Here's the drawing with two shaded views (mm, measured from the low corner). I have some questions. A direction names the side the tool comes from. Give positions to 0.01 mm unless a question says otherwise; leave off trailing zeros. Write each loop counter-clockwise with the first axis right and the second up, starting at its lowest first coordinate (ties: lowest second). Pieces come first, ordered by that corner, then holes.
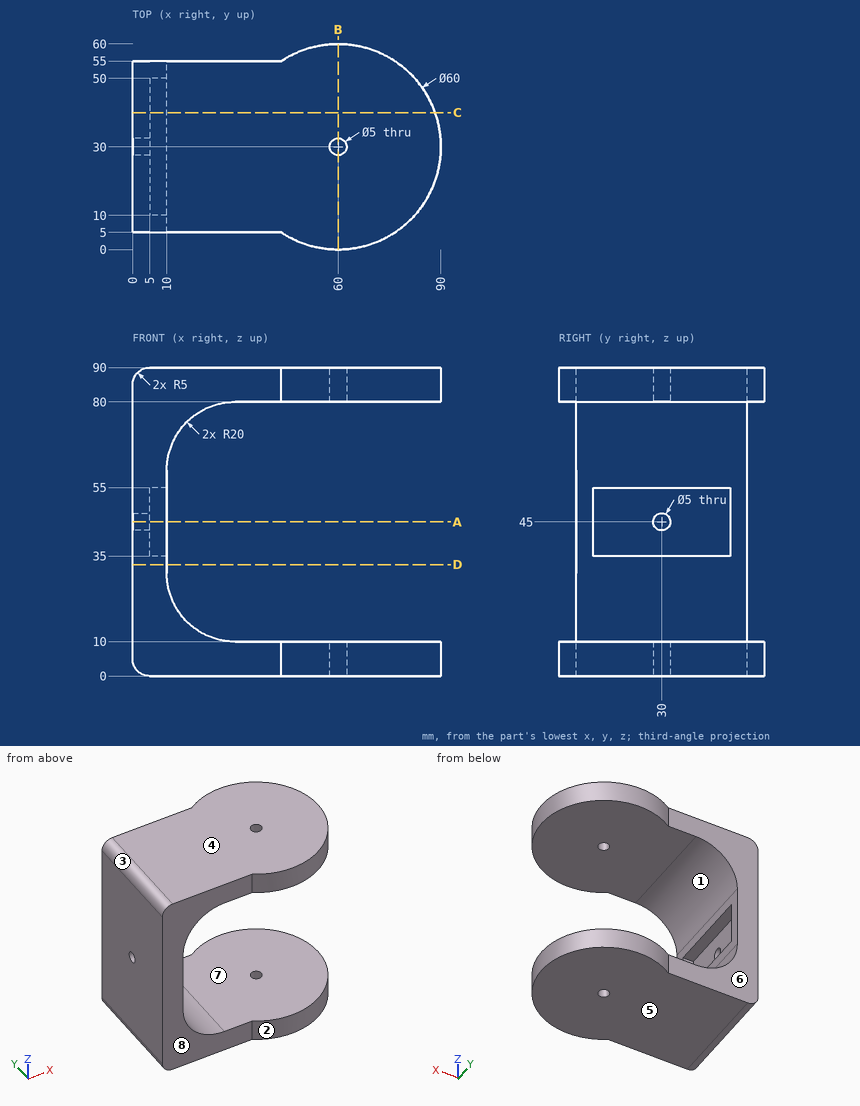
(1) Will these pins go through, and if not, where does the flat tip stop? P1, Ø22, axis at y = 34, z = 46, coming from the +X side; P2, Ø5.5, axis at x = 8, z = 42.5, coming from the -Y side; P3, Ø12, axis at x = 42, z = 11, coming from the -Y side.
Returned:
P1: stops at x = 10
P2: stops at y = 5
P3: stops at y = 2.54
(2) Imagine slicing it at B-B, the plane x = 60. Write out the boundary of the cut face in (y, z).
Returned:
outline: (0, 0) - (27.5, 0) - (27.5, 10) - (0, 10) - close; (0, 80) - (27.5, 80) - (27.5, 90) - (0, 90) - close; (32.5, 0) - (60, 0) - (60, 10) - (32.5, 10) - close; (32.5, 80) - (60, 80) - (60, 90) - (32.5, 90) - close
(3) Imagine slicing it at D-D, the plane z = 32.5. Write out the boundary of the cut face in (x, y).
Returned:
outline: (0, 5) - (10, 5) - (10, 55) - (0, 55) - close
(4) For the marked faces 4, 5, 6, 7 and 8, which set-ups out of +Z, -Z, +X, -X, +Y, -Y let a thin tool reach every point of the face, with its end or its side?
Returned:
face 4: +Z, +X, -X, +Y, -Y
face 5: -Z, +X, -X, +Y, -Y
face 6: +Z, -Z, -X, +Y
face 7: +X, +Y, -Y
face 8: +Z, -Z, -X, -Y
(5) If we mould it in two halves opening along Z, with no side actions, what happens to the marked faces 1, 2 and 3? For each: +Z half, -Z half, draft (parallel to the pull), parting line (faces both ways), or undercut.
Returned:
face 1: undercut
face 2: draft
face 3: +Z half
(6) If I drill on L1, parallel to Z at x = 67, y = 32; L2, parallel to Y at x = 2, z = 45; L3, parallel to Y at x = 60, z = 83, over which ranges is the centre line in solid material (lowest first)?
Returned:
L1: z = 0 to 10, 80 to 90
L2: y = 5 to 27.5, 32.5 to 55
L3: y = 0 to 27.5, 32.5 to 60
(7) Imagine slicing it at A-A, the plane z = 45. Write out the boundary of the cut face in (x, y), plus the area to 3 significant figures.
Returned:
outline: (0, 5) - (10, 5) - (10, 10) - (5, 10) - (5, 27.5) - (0, 27.5) - close; (0, 32.5) - (5, 32.5) - (5, 50) - (10, 50) - (10, 55) - (0, 55) - close
area: 275 mm2
(8) Imagine slicing it at C-C, the plane y = 40. Write out the boundary of the cut face in (x, z).
Returned:
outline: (0, 5) arc R5 ccw to (5, 0) - (88.28, 0) - (88.28, 10) - (30, 10) arc R20 cw to (10, 30) - (10, 35) - (5, 35) - (5, 55) - (10, 55) - (10, 60) arc R20 cw to (30, 80) - (88.28, 80) - (88.28, 90) - (5, 90) arc R5 ccw to (0, 85) - close
